Verification items for the finished model (mm, model axes). A direction names the side the tool comes from. Give positions to 0.01 mm unless a question says otherwise; leave off trailing zeros. Write each loop counter-clockwise with the first axis right and the second up, starting at its lowest first coordinate (ties: lowest second). Pieces come first, ordered by that corner, then holes. Notation, with made-up numbers: (83.25, -19.5) -> (130.25, -19.5) arc R17 cw to (130.25, -12.5) -> close; hole circle Ø4 at (36, -33.5). An arc over 180 degrees is marked (long way). Answer as CSV lines item,"result".
```python
from build123d import *

# Parameters (mm, degrees)
F1_DEPTH = 35.56
F3_DEPTH = 6.35
F5_DEPTH = 12.7
F6_W     = 50.8
F6_H     = 406.4
F7_DEPTH = 162.56


with BuildPart() as f1:
    # F0 (on Front) → F1 (new body)
    with BuildSketch(Plane.XZ):
        Polygon((-254, 152.4), (254, 152.4), (330.2, 152.4), (330.2, 203.2), (-330.2, 203.2), (-330.2, -203.2), (330.2, -203.2), (330.2, -152.4), (254, -152.4), (-254, -152.4), align=None)
    extrude(amount=F1_DEPTH)

    # F2 (on face) + F1_face (on face) → F3 (join)
    with BuildSketch(Plane(origin=(0, 0, 0), x_dir=(-1, 0, 0), z_dir=(0, 1, 0))):
        Polygon((254, 152.4), (-330.2, 152.4), (-330.2, 139.7), (241.3, 139.7), (241.3, -139.7), (-330.2, -139.7), (-330.2, -152.4), (254, -152.4), align=None)
        Polygon((330.2, 203.2), (-330.2, 203.2), (-330.2, 152.4), (254, 152.4), (254, -152.4), (-330.2, -152.4), (-330.2, -203.2), (330.2, -203.2), align=None)
    with BuildSketch(Plane(origin=(-75.111429, 0, 0), x_dir=(1, 0, 0), z_dir=(0, 1, 0))):
        Polygon((-178.888571, -152.4), (405.311429, -152.4), (405.311429, -203.2), (-255.088571, -203.2), (-255.088571, 203.2), (405.311429, 203.2), (405.311429, 152.4), (-178.888571, 152.4), align=None)
    extrude(amount=F3_DEPTH)

    # F4 (on face) → F5 (join)
    with BuildSketch(Plane.XZ.offset(35.56)):
        Polygon((330.2, 203.2), (-330.2, 203.2), (-330.2, -203.2), (330.2, -203.2), (330.2, -152.4), (-254, -152.4), (-254, 152.4), (330.2, 152.4), align=None)
        Polygon((330.2, 139.7), (330.2, 152.4), (-254, 152.4), (-254, -152.4), (330.2, -152.4), (330.2, -139.7), (-241.3, -139.7), (-241.3, 139.7), align=None)
    extrude(amount=F5_DEPTH)

    # F6 (on face) → F7 (cut)
    with BuildSketch(Plane(origin=(0, 6.35, 0), x_dir=(-1, 0, 0), z_dir=(0, 1, 0))):
        with Locations((-304.8, 0)):
            Rectangle(F6_W, F6_H)
    extrude(amount=-F7_DEPTH, mode=Mode.SUBTRACT)


solid = f1.part
```
1) Depth check by flat-ended pin: pin 1 (1.9 mm diameter, centred on y = 2.5, z = 36, fed in from +X). Enter the tip coordinate at first touch or a pass-through.
Reported:
pin 1,"x = -241.3"
2) Section check B-B (y = -16). Record the boundary of the cut face in (x, z).
Reported:
outline,"(-330.2, -203.2) -> (279.4, -203.2) -> (279.4, -152.4) -> (-254, -152.4) -> (-254, 152.4) -> (279.4, 152.4) -> (279.4, 203.2) -> (-330.2, 203.2) -> close"
3) Draft check along Z on faces 4 (the flat face through (-241.3, -42, -2)), 5 (the flat face through (279.4, -21, -179)), 6 (the flat face through (-68, -35.56, -146)), 7 (the flat face through (-30, -21, -203.2)). Enter one of: +Z half, -Z half, draft (parallel to the pull), parting line (faces both ways), or undercut.
Reported:
face 4,"undercut"
face 5,"draft"
face 6,"undercut"
face 7,"-Z half"
4) Tool access check on faces 1 (the flat face through (-254, -18, -2)), 2 (the flat face through (-21, -21, 203.2)), 3 (the flat face through (23, -42, -139.7)). Record the directions out of +Z, -Z, +X, -X, +Y, -Y that give a thin tool (end or side, any length) a straight path to the whole face; none if there is none.
Reported:
face 1,"+X"
face 2,"+Z, +X, -X, +Y, -Y"
face 3,"+X, +Y, -Y"
5) Section check A-A (x = 167). Record the boundary of the cut face in (y, z).
Reported:
outline,"(-48.26, -203.2) -> (6.35, -203.2) -> (6.35, -139.7) -> (0, -139.7) -> (0, -152.4) -> (-35.56, -152.4) -> (-35.56, -139.7) -> (-48.26, -139.7) -> close; (-48.26, 139.7) -> (-35.56, 139.7) -> (-35.56, 152.4) -> (0, 152.4) -> (0, 139.7) -> (6.35, 139.7) -> (6.35, 203.2) -> (-48.26, 203.2) -> close"
6) Scan lines: line 1 along Z through (x, y) = (150, -41); line 2 along Z through (x, y) = (-176, -12); line 3 along X through (y, z) = (-2, 151.5). Record each from-to range of solid material in increasing order.
Reported:
line 1,"-203.2 to -139.7, 139.7 to 203.2"
line 2,"-203.2 to -152.4, 152.4 to 203.2"
line 3,"-330.2 to -254"
7) Section check C-C (z = 22.5). Record the boundary of the cut face in (x, y), and give its area (3 significant figures).
Reported:
outline,"(-330.2, -48.26) -> (-241.3, -48.26) -> (-241.3, -35.56) -> (-254, -35.56) -> (-254, 0) -> (-241.3, 0) -> (-241.3, 6.35) -> (-330.2, 6.35) -> close"
area,"4,400 mm²"
